```python
from build123d import *

# Parameters (mm, degrees)
F0_W     = 47.5
F0_H     = 47.5
F1_DEPTH = 20
F2_DEPTH = 15
F4_DEPTH = 20.001


with BuildPart() as f1:
    # F0 (on Front) → F1 (new body)
    with BuildSketch(Plane.XZ):
        Rectangle(F0_W, F0_H)
        Polygon((0, 19.7989898732), (19.7989898732, 19.7989898732), (19.7989898732, 0), (19.7989898732, -19.7989898732), (0, -19.7989898732), (-19.7989898732, -19.7989898732), (-19.7989898732, 0), (-19.7989898732, 19.7989898732), align=None, mode=Mode.SUBTRACT)
        Polygon((-19.7989898732, 0), (0, 19.7989898732), (-19.7989898732, 19.7989898732), align=None)
        Polygon((0, -19.7989898732), (-19.7989898732, 0), (-19.7989898732, -19.7989898732), align=None)
        Polygon((19.7989898732, -19.7989898732), (19.7989898732, 0), (0, -19.7989898732), align=None)
        Polygon((19.7989898732, 0), (19.7989898732, 19.7989898732), (0, 19.7989898732), align=None)
    extrude(amount=F1_DEPTH)

    # F2 (add): a face of the model
    f2_faces = [f1.faces().sort_by_distance(p)[0] for p in [
        (0, -10, 23.75),
    ]]
    extrude(f2_faces, amount=F2_DEPTH)

    # F3 (on face) → F4 (cut, through all)
    with BuildSketch(Plane.XZ.offset(20)):
        Polygon((-23.75, 38.75), (-23.75, 0), (-7.5, 38.75), align=None)
        Polygon((23.75, 38.75), (7.5, 38.75), (23.75, 0), align=None)
    extrude(amount=-F4_DEPTH, mode=Mode.SUBTRACT)


solid = f1.part
```
Can you work these out from the model? Positions are in its coordinate system, mm. A direction names the side the tool comes from. Give positions to 0.01 mm unless a question says otherwise; leave off trailing zeros. Loops run counter-clockwise (first coordinate to the right, second up) from the corner with the lowest first, then second, coordinate; pieces in that order, holes last. Notation, with made-up numbers: M -15,-7 L -2,-7 A19 ccw -2,3 Z; hole C 19,51 d5. An arc over 180 degrees is marked long. One line per item, written item: value.
(1) Suppose I cut it at C-C on z = -14. List the corners of the cut face in (x, y) for me, plus the area to 3 significant figures.
Returned:
outline: M -23.75,-20 L -5.8,-20 L -5.8,0 L -23.75,0 Z; M 5.8,-20 L 23.75,-20 L 23.75,0 L 5.8,0 Z
area: 718 mm^2
(2) Which directions (+Z, -Z, +X, -X, +Y, -Y) give clear straight access to the entire face, cutting with the end or side of a thin tool? Please do faces 5 (the face through (-9.8, -9.9, -10)), 6 (the face through (10, 0, 14)).
Returned:
face 5: +Y, -Y
face 6: +Z, -Z, +X, -X, +Y
(3) Suppose I cut it at B-B on x = 16. List the corners of the cut face in (y, z) for me, plus the area to 3 significant figures.
Returned:
outline: M -20,-23.75 L 0,-23.75 L 0,-3.8 L -20,-3.8 Z; M -20,3.8 L 0,3.8 L 0,18.48 L -20,18.48 Z
area: 693 mm^2
(4) Suppose I cut it at D-D on z = 21. List the corners of the cut face in (x, y) for me.
Returned:
outline: M -14.94,-20 L 14.94,-20 L 14.94,0 L -14.94,0 Z
(5) Will these pins go through, and if not, where does the flat tip stop? pin 1 (12 mm diameter, centred on y = -12.5, z = 26.5, fed in from -X); pin 2 (6 mm diameter, centred on x = 18.5, y = -3.5, fed in from +Z).
Returned:
pin 1: x = -15.15
pin 2: z = 19.67
(6) Suppose I cut it at A-A on y = -13.5. List the corners of the cut face in (x, z) for me, plus the area to 3 significant figures.
Returned:
outline: M -23.75,-23.75 L 23.75,-23.75 L 23.75,0 L 7.5,38.75 L -7.5,38.75 L -23.75,0 Z; hole M -19.8,0 L 0,-19.8 L 19.8,0 L 0,19.8 Z
area: 1,560 mm^2
(7) I need wall thicknesses on line 1 (Z direction, x = -4.5, y = -2); line 2 (X direction, y = -5, z = -7); line 3 (Z direction, x = 13, y = -3.5). Which ranges of each line are inside material? Lowest first, please.
Returned:
line 1: -23.75 to -15.3, 15.3 to 38.75
line 2: -23.75 to -12.8, 12.8 to 23.75
line 3: -23.75 to -6.8, 6.8 to 25.63
(8) We'd pull the mould along X, two halves only. Please class faces 1 (the face through (-10, -9.9, 9.8)), 2 (the face through (23.75, -10, -12)), 3 (the face through (0, -10, 38.75)), 4 (the face through (-23.75, -10, -12)): released by +X, released by -X, zero draft, split by the parting line, or undercut.
Returned:
face 1: undercut
face 2: released by +X
face 3: zero draft
face 4: released by -X
